Input: part model. Units: mm. Frame: model coordinates. A direction names the side the tool comes from. Coordinates: 2 decimals unless noted, no trailing zeros. Order: outer loops, then holes, each group sorted by start corner. A loop starts at its lowest first (then second) coordinate and runs counter-clockwise, first axis right, second up. Notation, with made-up numbers: (-6.75, 66.5) - (20.25, 66.5) arc R22 ccw to (20.25, 89.5) - close; hole circle Ø2 at (58, -4.75). An arc over 180 degrees is marked (long way). One line per question, with ' | ' between items.
from build123d import *

# Parameters (mm, degrees)
ESQUISSE2_W                  = 27.2
ESQUISSE2_H                  = 14.017263762
BOSS_EXTRU_1_DEPTH           = 10
ESQUISSE3_R                  = 1.6
ENL_V_MAT_EXTRU_1_DEPTH      = 69.128187999
R_P_TITION_CIRCULAIRE1_COUNT = 3


with BuildPart() as part:
    # Esquisse1 → R_volution1 (revolve)
    with BuildSketch(Plane.XY, mode=Mode.PRIVATE) as r_volution1_sk:
        Polygon((-6, 0), (-12, 0), (-27, 30.3), (-27, 40.3), (-22, 40.3), (-22, 33.237189942), (-6, 7.254793936), align=None)
    revolve(r_volution1_sk.sketch.rotate(Axis((0, 0, 0), (0, 1, 0)), 270), axis=Axis((0, 0, 0), (0, 1, 0)))

    # Esquisse2 → Boss.-Extru.1 (add)
    with BuildSketch(Plane(origin=(0, 40.3, 0), x_dir=(1, 0, 0), z_dir=(0, 1, 0))):
        with Locations((0, 29.991368119)):
            Rectangle(ESQUISSE2_W, ESQUISSE2_H)
    boss_extru_1 = extrude(amount=-BOSS_EXTRU_1_DEPTH)

    # Esquisse3 → Enl_v. mat.-Extru.1 (cut, through all)
    with BuildSketch(Plane.ZY.offset(13.6)):
        with Locations((-32, 35.3)):
            Circle(ESQUISSE3_R)
    enl_v_mat_extru_1 = extrude(amount=-ENL_V_MAT_EXTRU_1_DEPTH, mode=Mode.SUBTRACT)

    # R_p_tition circulaire1: Boss.-Extru.1, Enl_v. mat.-Extru.1 ×3 about axis
    r_p_tition_circulaire1_axis = Axis((0, 0, 0), (0, 1, 0))
    add([boss_extru_1.rotate(r_p_tition_circulaire1_axis, i * 360 / R_P_TITION_CIRCULAIRE1_COUNT) for i in range(1, R_P_TITION_CIRCULAIRE1_COUNT)])
    add([enl_v_mat_extru_1.rotate(r_p_tition_circulaire1_axis, i * 360 / R_P_TITION_CIRCULAIRE1_COUNT) for i in range(1, R_P_TITION_CIRCULAIRE1_COUNT)], mode=Mode.SUBTRACT)


solid = part.part
Item 1: Section D-D on y = 15. Return the cut outline in (x, z).
Data:
outline: circle Ø38.85 at (0, 0); hole circle Ø21.54 at (0, 0)
Item 2: Section C-C on y = 35.3. Return the cut outline in (x, z), and give its area (3 significant figures).
Data:
outline: (-38.84, 6.72) - (-35.9, 5.02) - (-22.3, 28.58) - (-25.24, 30.28) - close; (-33.13, 3.42) - (-27, -0.12) arc R27 ccw to (-13.6, -23.32) - (-13.6, -30.4) - (13.6, -30.4) - (13.6, -23.32) arc R27 ccw to (27, -0.12) - (33.13, 3.42) - (19.53, 26.98) - (13.4, 23.44) arc R27 ccw to (-13.4, 23.44) - (-19.53, 26.98) - close; (-13.6, -37) - (13.6, -37) - (13.6, -33.6) - (-13.6, -33.6) - close; (22.3, 28.58) - (35.9, 5.02) - (38.84, 6.72) - (25.24, 30.28) - close; hole circle Ø44 at (0, 0) | area: 1,420 mm^2
Item 3: Section B-B on z = -32. Return the cut outline in (x, y), and give its area (3 significant figures).
Data:
outline: (-13.6, 30.3) - (13.6, 30.3) - (13.6, 33.7) - (-13.6, 33.7) - close; (-13.6, 36.9) - (13.6, 36.9) - (13.6, 40.3) - (-13.6, 40.3) - close | area: 185 mm^2
Item 4: Access query for faces 4 (the face through (-19.24, 35.37, 26.81)), 5 (the face through (21.477, 36.719, 4.769)), 6 (the face through (-13.6, 35, -30)), 7 (the face through (28, 30.3, 16)). Directions: +Z, -Z, +X, -X, +Y, -Y. A direction counts if a zero-diameter tool reaches every point of the face in a straight line with its end or side. Return the directions, or none.
Data:
face 4: +Z, +Y, -Y | face 5: +Y | face 6: -Z, -X, +Y, -Y | face 7: +Z, +X, -Y
Item 5: Ray query, line 1 (Y direction, x = -0.25, z = -32); line 2 (X direction, y = 4, z = 0); line 3 (Y direction, x = -11, z = -31.5). Return the intervals inside material, ascending.
Data:
line 1: 30.3 to 33.7, 36.9 to 40.3 | line 2: -13.98 to -6, 6 to 13.98 | line 3: 30.3 to 33.78, 36.82 to 40.3
Item 6: Draft query along X for faces 1 (the face through (-32.838, 35.37, 3.255)), 2 (the face through (23.48, 35.37, -13.33)), 3 (the face through (-1.802, 3.577, -5.723)). Return one class per face: released by +X, released by -X, zero draft, split by the parting line, or undercut.
Data:
face 1: released by -X | face 2: released by +X | face 3: undercut
Item 7: Contact query for flat-ended pins moving along their axis: P1, Ø4, axis at x = 2, z = -23, coming from the -Y side; P2, Ø1.5, axis at y = 24, z = -14, coming from the +X side; P3, Ø5, axis at y = 36.5, z = -32, coming from the -X side. Output: stop coordinate, or through.
Data:
P1: y = 18.36 | P2: x = 20.04 | P3: x = -13.6
Item 8: Section A-A on x = 0. Return the cut outline in (y, z), and give its area (3 significant figures).
Data:
outline: (0, -12) - (30.3, -27) - (30.3, -37) - (40.3, -37) - (40.3, -22) - (33.24, -22) - (7.25, -6) - (0, -6) - close; (0, 6) - (7.25, 6) - (33.24, 22) - (40.3, 22) - (40.3, 27) - (30.3, 27) - (0, 12) - close; hole circle Ø3.2 at (35.3, -32) | area: 688 mm^2
